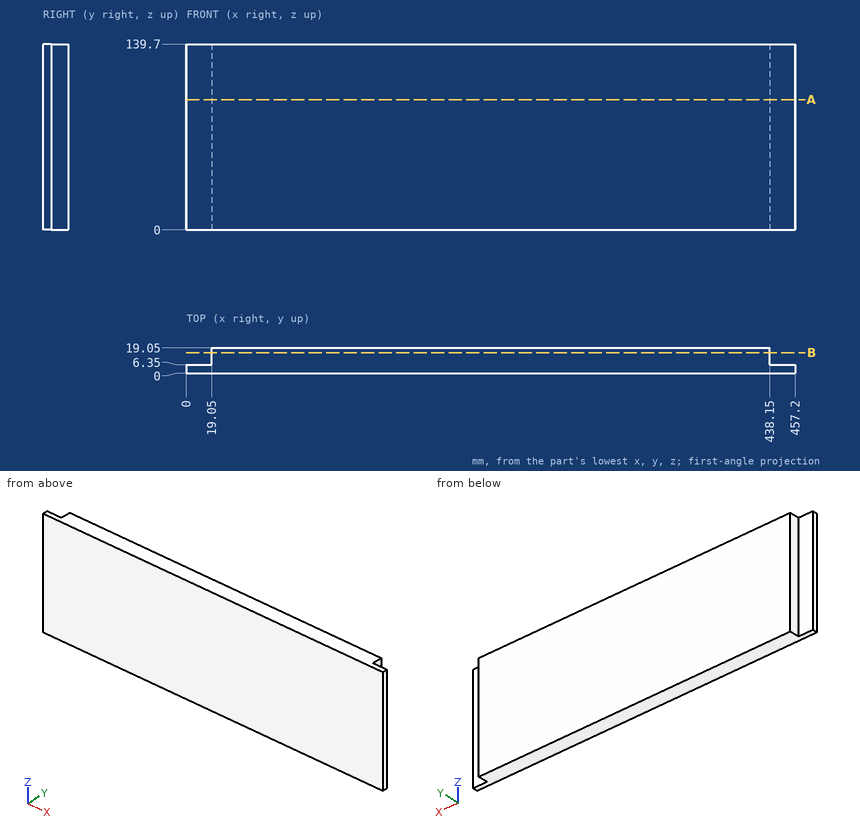
Drawing for the job (mm, zero at the part's lowest x, y, z). Round coordinates to 2 decimals unless told otherwise and drop trailing zeros. Order: outer loops, then holes, each group sorted by start corner. A loop starts at its lowest first (then second) coordinate and runs counter-clockwise, first axis right, second up. Notation, with made-up numbers: (8.25, 10.5) -> (55.25, 10.5) arc R8 ccw to (55.25, 25.5) -> close; hole circle Ø11 at (0, 41.25). An arc over 180 degrees is marked (long way). Write item = value, one per line. Start each with the question number.
(1) Cut at A-A, the plane z = 98. List the corners of the cut face in (x, y), then the cut area to 3 significant figures.
(2) Probe line 1 (X direction, y = 15.5, z = 54.5). List the from-to ranges inside material, lowest first. Write a range as [from, to].
(3) Cut at B-B, the plane y = 15.5. List the corners of the cut face in (x, z).
(4) Pin check, flat tips, straight feed: P1, Ø8, axis at y = 13.5, z = 37.5, coming from the -X side; P2, Ø15, axis at x = 11, z = 45, coming from the +Y side. Stop position of each tip, or through.
Model answer:
q1.outline = (0, 0) -> (457.2, 0) -> (457.2, 6.35) -> (438.15, 6.35) -> (438.15, 19.05) -> (19.05, 19.05) -> (19.05, 6.35) -> (0, 6.35) -> close
q1.area = 8,230 mm2
q2.line_1 = [19.05, 438.15]
q3.outline = (19.05, 0) -> (438.15, 0) -> (438.15, 139.7) -> (19.05, 139.7) -> close
q4.P1 = 19.05
q4.P2 = 6.35
